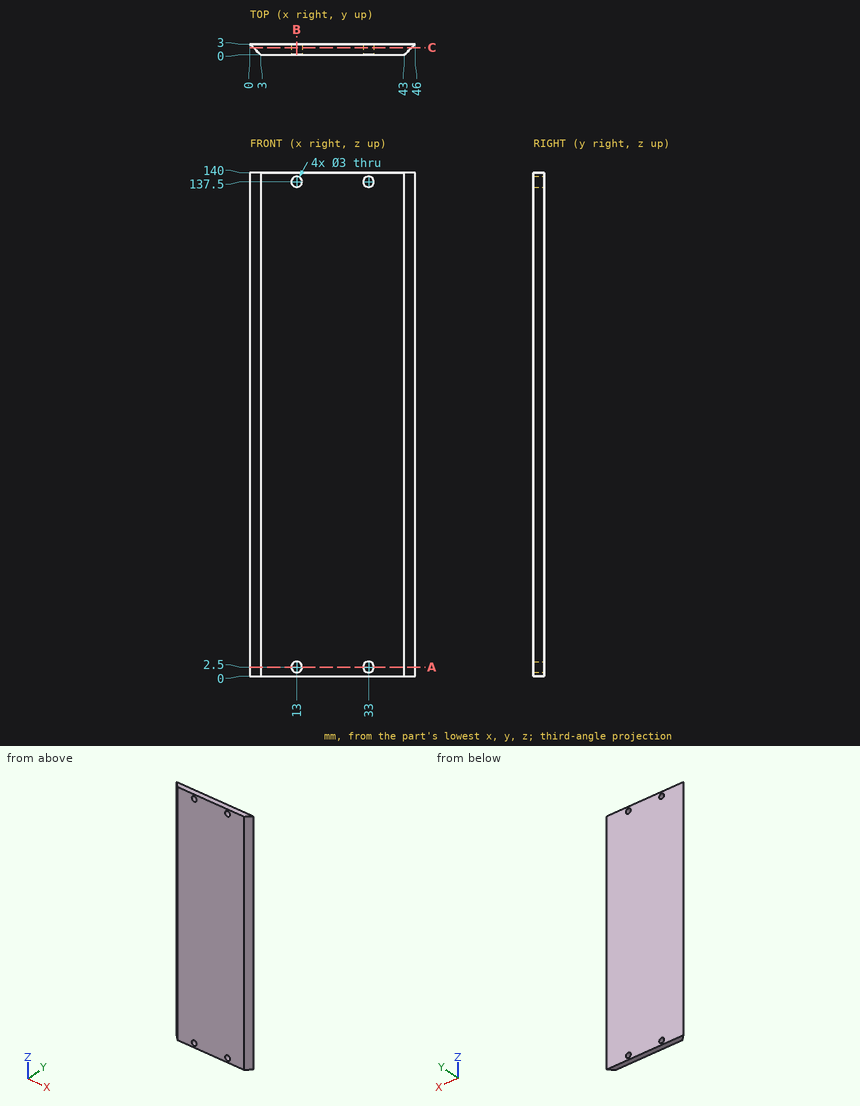
Here's the drawing with two shaded views (mm, measured from the low corner). I have some questions. Coordinates: 2 decimals unless noted, no trailing zeros. Order: outer loops, then holes, each group sorted by start corner. A loop starts at its lowest first (then second) coordinate and runs counter-clockwise, first axis right, second up. Notation, with made-up numbers: (77.5, 64.25) - (127.5, 64.25) arc R26 cw to (127.5, 97.25) - close; hole circle Ø7 at (39, 68). An arc over 180 degrees is marked (long way). Answer in a Markdown table with one row per item.
1. If I drill on line 1 along Z through (x, y) = (34, 0.9); line 2 along X through (y, z) = (0.7, 2.5); line 3 along Y through (x, z) = (44, 79.5), over which ranges is the centre line in solid material (lowest first)?
Reply:
| item | result |
|---|---|
| line 1 | z = 0 to 1.38, 3.62 to 136.38, 138.62 to 140 |
| line 2 | x = 2.3 to 11.5, 14.5 to 31.5, 34.5 to 43.7 |
| line 3 | y = 1 to 3 |
2. Suppose I cut it at A-A (z = 2.5). Please give me the cut outline in (x, y), and give its area (3 significant figures).
Reply:
| item | result |
|---|---|
| outline | (0, 3) - (3, 0) - (11.5, 0) - (11.5, 3) - close; (14.5, 0) - (31.5, 0) - (31.5, 3) - (14.5, 3) - close; (34.5, 0) - (43, 0) - (46, 3) - (34.5, 3) - close |
| area | 111 mm^2 |
3. For pin 1 (1 mm diameter, centred on y = 1.5, z = 113, fed in from +X); pin 2 (5 mm diameter, centred on x = 33, z = 137.5, fed in from -Y), each with a flat end and sliding along its axis, tell me the tip position at first contact or that it passes through.
Reply:
| item | result |
|---|---|
| pin 1 | stops at x = 45 |
| pin 2 | stops at y = 0 |
4. Suppose I cut it at C-C (y = 2). Please give me the cut outline in (x, z).
Reply:
| item | result |
|---|---|
| outline | (1, 0) - (45, 0) - (45, 140) - (1, 140) - close; hole circle Ø3 at (13, 2.5); hole circle Ø3 at (13, 137.5); hole circle Ø3 at (33, 2.5); hole circle Ø3 at (33, 137.5) |
5. Suppose I cut it at B-B (x = 13). Please give me the cut outline in (y, z).
Reply:
| item | result |
|---|---|
| outline | (0, 0) - (3, 0) - (3, 1) - (0, 1) - close; (0, 4) - (3, 4) - (3, 136) - (0, 136) - close; (0, 139) - (3, 139) - (3, 140) - (0, 140) - close |
